Build history of the part. All positions in model axes, mm. A direction names the side the tool comes from. Give positions to 0.01 mm unless a question says otherwise; leave off trailing zeros. Order: outer loops, then holes, each group sorted by start corner. A loop starts at its lowest first (then second) coordinate and runs counter-clockwise, first axis right, second up. Notation, with made-up numbers: (35.5, 66) - (83.5, 66) arc R18 ccw to (83.5, 73) - close; hole circle Ø3 at (64, -10). An arc over 180 degrees is marked (long way). Write each question's results on one line, items separated by ' | '. Start each with the question number.
1) Two-plate mould, pull along X, no slides. Class faces 1 (the face through (146.39, 4.06, 206.58)), 2 (the face through (-150, 4, -9)), 3 (the face through (38.58, 4.06, -93.61)): +X half, -X half, draft (parallel to the pull), parting line (faces both ways), or undercut.
2) Drill centre lines: line 1 along X through (y, z) = (6.25, 199); line 2 along X through (y, z) = (4.5, 156); line 3 along X through (y, z) = (6, -113). Where is each one in solid material? Low to high. Write a range as from..to.
3) Cut at B-B on x = -95. List the corners of the cut face in (y, z), plus the area to 3 significant figures.
4) Cut at C-C on x = -10.5. List the corners of the cut face in (y, z), plus the area to 3 significant figures.
5) Cut at A-A on z = -149.5. List the corners of the cut face in (x, y).
6) Cut at D-D on y = 3.5. State how many separate pieces and enclosed holes the cut face has, plus the area to 3 significant figures.
7) Drop a flat-ended pin along its axis: pin 1 Ø2.5 at (x, z) = (137, 43) entering from -Y. Give the stop position or say it passes through.
8) Tool access for faces 4 (the face through (-45.61, 4.06, -206.58)), 5 (the face through (113.559, 3.944, -130.796)): list every direction of +Z, -Z, +X, -X, +Y, -Y with a clear straight run to the whole face (end or side of a thin tool).
from build123d import *

# Parameters (mm, degrees)
SKETCH1_R           = 2.5
SKETCH1_R_2         = 1.5
SKETCH1_R_3         = 30.5
BOSS_EXTRUDE1_DEPTH = 8
FILLET1_R           = 12


with BuildPart() as part:
    # Sketch1 → Boss-Extrude1 (new body)
    with BuildSketch(Plane(origin=(0, 0, 0), x_dir=(1, 0, 0), z_dir=(0, 1, 0))):
        Polygon((-150, -210), (150, -210), (150, 210), (42, 210), (42, 90), (0, 90), (-42, 90), (-42, 210), (-150, 210), align=None)
        with Locations(Location((-21, 78, 0), (0, 0, 270))):
            Circle(SKETCH1_R, mode=Mode.SUBTRACT)
        with Locations(Location((21, 78, 0), (0, 0, 90))):
            Circle(SKETCH1_R, mode=Mode.SUBTRACT)
        with Locations(Location((-28.5, -138, 0), (0, 0, 270))):
            Circle(SKETCH1_R_2, mode=Mode.SUBTRACT)
        with Locations(Location((-28.5, -162, 0), (0, 0, 270))):
            Circle(SKETCH1_R_2, mode=Mode.SUBTRACT)
        with Locations(Location((-28.5, -186, 0), (0, 0, 270))):
            Circle(SKETCH1_R_2, mode=Mode.SUBTRACT)
        with Locations(Location((28.5, -186, 0), (0, 0, 90))):
            Circle(SKETCH1_R_2, mode=Mode.SUBTRACT)
        with Locations(Location((28.5, -162, 0), (0, 0, 90))):
            Circle(SKETCH1_R_2, mode=Mode.SUBTRACT)
        with Locations(Location((28.5, -138, 0), (0, 0, 90))):
            Circle(SKETCH1_R_2, mode=Mode.SUBTRACT)
        with Locations(Location((-95, 155, 0), (0, 0, 270))):
            Circle(SKETCH1_R_3, mode=Mode.SUBTRACT)
        with Locations(Location((-137, 197, 0), (0, 0, 270))):
            Circle(SKETCH1_R_2, mode=Mode.SUBTRACT)
        with Locations(Location((-53, 197, 0), (0, 0, 270))):
            Circle(SKETCH1_R_2, mode=Mode.SUBTRACT)
        with Locations(Location((-53, 113, 0), (0, 0, 270))):
            Circle(SKETCH1_R_2, mode=Mode.SUBTRACT)
        with Locations(Location((-137, 113, 0), (0, 0, 270))):
            Circle(SKETCH1_R_2, mode=Mode.SUBTRACT)
        with Locations(Location((-137, 35, 0), (0, 0, 270))):
            Circle(SKETCH1_R_2, mode=Mode.SUBTRACT)
        with Locations(Location((-137, -43, 0), (0, 0, 270))):
            Circle(SKETCH1_R_2, mode=Mode.SUBTRACT)
        with Locations(Location((-137, -121, 0), (0, 0, 270))):
            Circle(SKETCH1_R_2, mode=Mode.SUBTRACT)
        with Locations(Location((137, -121, 0), (0, 0, 90))):
            Circle(SKETCH1_R_2, mode=Mode.SUBTRACT)
        with Locations(Location((137, -43, 0), (0, 0, 90))):
            Circle(SKETCH1_R_2, mode=Mode.SUBTRACT)
        with Locations(Location((137, 35, 0), (0, 0, 90))):
            Circle(SKETCH1_R_2, mode=Mode.SUBTRACT)
        with Locations(Location((53, 197, 0), (0, 0, 90))):
            Circle(SKETCH1_R_2, mode=Mode.SUBTRACT)
        with Locations(Location((137, 197, 0), (0, 0, 90))):
            Circle(SKETCH1_R_2, mode=Mode.SUBTRACT)
        with Locations(Location((137, 113, 0), (0, 0, 90))):
            Circle(SKETCH1_R_2, mode=Mode.SUBTRACT)
        with Locations(Location((95, 155, 0), (0, 0, 90))):
            Circle(SKETCH1_R_3, mode=Mode.SUBTRACT)
        with Locations(Location((53, 113, 0), (0, 0, 90))):
            Circle(SKETCH1_R_2, mode=Mode.SUBTRACT)
        with Locations(Location((-53, 35, 0), (0, 0, 270))):
            Circle(SKETCH1_R_2, mode=Mode.SUBTRACT)
        with Locations(Location((-53, -43, 0), (0, 0, 270))):
            Circle(SKETCH1_R_2, mode=Mode.SUBTRACT)
        with Locations(Location((-53, -121, 0), (0, 0, 270))):
            Circle(SKETCH1_R_2, mode=Mode.SUBTRACT)
        with Locations(Location((53, -121, 0), (0, 0, 90))):
            Circle(SKETCH1_R_2, mode=Mode.SUBTRACT)
        with Locations(Location((53, -43, 0), (0, 0, 90))):
            Circle(SKETCH1_R_2, mode=Mode.SUBTRACT)
        with Locations(Location((53, 35, 0), (0, 0, 90))):
            Circle(SKETCH1_R_2, mode=Mode.SUBTRACT)
        with Locations(Location((-137, -199, 0), (0, 0, 270))):
            Circle(SKETCH1_R_2, mode=Mode.SUBTRACT)
        with Locations(Location((137, -199, 0), (0, 0, 90))):
            Circle(SKETCH1_R_2, mode=Mode.SUBTRACT)
        with Locations(Location((-120, -192, 0), (0, 0, 270))):
            Circle(SKETCH1_R_2, mode=Mode.SUBTRACT)
        with Locations(Location((-48, -192, 0), (0, 0, 270))):
            Circle(SKETCH1_R_2, mode=Mode.SUBTRACT)
        with Locations(Location((-48, -156, 0), (0, 0, 270))):
            Circle(SKETCH1_R_2, mode=Mode.SUBTRACT)
        with Locations(Location((-120, -156, 0), (0, 0, 270))):
            Circle(SKETCH1_R_2, mode=Mode.SUBTRACT)
        with Locations(Location((48, -156, 0), (0, 0, 90))):
            Circle(SKETCH1_R_2, mode=Mode.SUBTRACT)
        with Locations(Location((48, -192, 0), (0, 0, 90))):
            Circle(SKETCH1_R_2, mode=Mode.SUBTRACT)
        with Locations(Location((120, -192, 0), (0, 0, 90))):
            Circle(SKETCH1_R_2, mode=Mode.SUBTRACT)
        with Locations(Location((120, -156, 0), (0, 0, 90))):
            Circle(SKETCH1_R_2, mode=Mode.SUBTRACT)
    extrude(amount=BOSS_EXTRUDE1_DEPTH)

    # Fillet1
    fillet1_edges = [part.edges().sort_by_distance(p)[0] for p in [
        (150, 4, 210),
        (-150, 4, 210),
        (-42, 4, -210),
        (-42, 4, -90),
        (42, 4, -90),
        (42, 4, -210),
    ]]
    fillet(fillet1_edges, radius=FILLET1_R)


solid = part.part
Results:
1) face 1: +X half | face 2: -X half | face 3: undercut
2) line 1: -149.96..-138.5, -135.5..135.5, 138.5..149.96 | line 2: -150..-121.5, -118.5..-49.5, -46.5..46.5, 49.5..118.5, 121.5..150 | line 3: -150..-138.5, -135.5..-54.5, -51.5..-42, 42..51.5, 54.5..135.5, 138.5..150
3) outline: (0, -210) - (8, -210) - (8, -185.5) - (0, -185.5) - close; (0, -124.5) - (8, -124.5) - (8, 210) - (0, 210) - close | area: 2,870 mm^2
4) outline: (0, -90) - (8, -90) - (8, 210) - (0, 210) - close | area: 2,400 mm^2
5) outline: (-150, 0) - (-125, 0) - (-125, 8) - (-150, 8) - close; (-65, 0) - (-42, 0) - (-42, 8) - (-65, 8) - close; (42, 0) - (65, 0) - (65, 8) - (42, 8) - close; (125, 0) - (150, 0) - (150, 8) - (125, 8) - close
6) separate pieces: 1 | enclosed holes: 40 | area: 110,000 mm^2
7) pin 1: through
8) face 4: -Z, +Y, -Y | face 5: +Y, -Y
